from build123d import *

# Parameters (mm, degrees)
BOSS_EXTRUDE4_DEPTH = 5
SKETCH10_R          = 2.5
CUT_EXTRUDE3_DEPTH  = 5


with BuildPart() as part:
    # Sketch9 → Boss-Extrude4 (new body)
    with BuildSketch(Plane.XY):
        with BuildLine():
            add(Edge.make_bspline(
                [(0, 26.124355653), (3.884864274, 23.788582221), (-1.912523876, 17.903903592), (4.641256317, 17.321404385)],
                knots=[0, 0, 0, 0, 1, 1, 1, 1], degree=3))
            add(Edge.make_bspline(
                [(13.062177826, 22.624355653), (8.529899959, 22.54394866), (10.608246058, 14.5489734), (4.641256317, 17.321404385)],
                knots=[0, 0, 0, 0, 1, 1, 1, 1], degree=3))
            add(Edge.make_bspline(
                [(13.062177826, 22.624355653), (15.258682262, 18.659084387), (7.295657534, 16.461497276), (12.680148068, 12.680148068)],
                knots=[0, 0, 0, 0, 1, 1, 1, 1], degree=3))
            add(Edge.make_bspline(
                [(22.624355653, 13.062177826), (18.659084387, 15.258682262), (16.461497276, 7.295657534), (12.680148068, 12.680148068)],
                knots=[0, 0, 0, 0, 1, 1, 1, 1], degree=3))
            add(Edge.make_bspline(
                [(22.624355653, 13.062177826), (22.54394866, 8.529899959), (14.5489734, 10.608246058), (17.321404385, 4.641256317)],
                knots=[0, 0, 0, 0, 1, 1, 1, 1], degree=3))
            add(Edge.make_bspline(
                [(26.124355653, 0), (23.788582221, 3.884864274), (17.903903592, -1.912523876), (17.321404385, 4.641256317)],
                knots=[0, 0, 0, 0, 1, 1, 1, 1], degree=3))
            add(Edge.make_bspline(
                [(26.124355653, 0), (23.788582221, -3.884864274), (17.903903592, 1.912523876), (17.321404385, -4.641256317)],
                knots=[0, 0, 0, 0, 1, 1, 1, 1], degree=3))
            add(Edge.make_bspline(
                [(22.624355653, -13.062177826), (22.54394866, -8.529899959), (14.5489734, -10.608246058), (17.321404385, -4.641256317)],
                knots=[0, 0, 0, 0, 1, 1, 1, 1], degree=3))
            add(Edge.make_bspline(
                [(22.624355653, -13.062177826), (18.659084387, -15.258682262), (16.461497276, -7.295657534), (12.680148068, -12.680148068)],
                knots=[0, 0, 0, 0, 1, 1, 1, 1], degree=3))
            add(Edge.make_bspline(
                [(13.062177826, -22.624355653), (15.258682262, -18.659084387), (7.295657534, -16.461497276), (12.680148068, -12.680148068)],
                knots=[0, 0, 0, 0, 1, 1, 1, 1], degree=3))
            add(Edge.make_bspline(
                [(13.062177826, -22.624355653), (8.529899959, -22.54394866), (10.608246058, -14.5489734), (4.641256317, -17.321404385)],
                knots=[0, 0, 0, 0, 1, 1, 1, 1], degree=3))
            add(Edge.make_bspline(
                [(0, -26.124355653), (3.884864274, -23.788582221), (-1.912523876, -17.903903592), (4.641256317, -17.321404385)],
                knots=[0, 0, 0, 0, 1, 1, 1, 1], degree=3))
            add(Edge.make_bspline(
                [(0, -26.124355653), (-3.884864274, -23.788582221), (1.912523876, -17.903903592), (-4.641256317, -17.321404385)],
                knots=[0, 0, 0, 0, 1, 1, 1, 1], degree=3))
            add(Edge.make_bspline(
                [(-13.062177826, -22.624355653), (-8.529899959, -22.54394866), (-10.608246058, -14.5489734), (-4.641256317, -17.321404385)],
                knots=[0, 0, 0, 0, 1, 1, 1, 1], degree=3))
            add(Edge.make_bspline(
                [(-13.062177826, -22.624355653), (-15.258682262, -18.659084387), (-7.295657534, -16.461497276), (-12.680148068, -12.680148068)],
                knots=[0, 0, 0, 0, 1, 1, 1, 1], degree=3))
            add(Edge.make_bspline(
                [(-22.624355653, -13.062177826), (-18.659084387, -15.258682262), (-16.461497276, -7.295657534), (-12.680148068, -12.680148068)],
                knots=[0, 0, 0, 0, 1, 1, 1, 1], degree=3))
            add(Edge.make_bspline(
                [(-22.624355653, -13.062177826), (-22.54394866, -8.529899959), (-14.5489734, -10.608246058), (-17.321404385, -4.641256317)],
                knots=[0, 0, 0, 0, 1, 1, 1, 1], degree=3))
            add(Edge.make_bspline(
                [(-26.124355653, 0), (-23.788582221, -3.884864274), (-17.903903592, 1.912523876), (-17.321404385, -4.641256317)],
                knots=[0, 0, 0, 0, 1, 1, 1, 1], degree=3))
            add(Edge.make_bspline(
                [(-26.124355653, 0), (-23.788582221, 3.884864274), (-17.903903592, -1.912523876), (-17.321404385, 4.641256317)],
                knots=[0, 0, 0, 0, 1, 1, 1, 1], degree=3))
            add(Edge.make_bspline(
                [(-22.624355653, 13.062177826), (-22.54394866, 8.529899959), (-14.5489734, 10.608246058), (-17.321404385, 4.641256317)],
                knots=[0, 0, 0, 0, 1, 1, 1, 1], degree=3))
            add(Edge.make_bspline(
                [(-22.624355653, 13.062177826), (-18.659084387, 15.258682262), (-16.461497276, 7.295657534), (-12.680148068, 12.680148068)],
                knots=[0, 0, 0, 0, 1, 1, 1, 1], degree=3))
            add(Edge.make_bspline(
                [(-13.062177826, 22.624355653), (-15.258682262, 18.659084387), (-7.295657534, 16.461497276), (-12.680148068, 12.680148068)],
                knots=[0, 0, 0, 0, 1, 1, 1, 1], degree=3))
            add(Edge.make_bspline(
                [(-13.062177826, 22.624355653), (-8.529899959, 22.54394866), (-10.608246058, 14.5489734), (-4.641256317, 17.321404385)],
                knots=[0, 0, 0, 0, 1, 1, 1, 1], degree=3))
            add(Edge.make_bspline(
                [(0, 26.124355653), (-3.884864274, 23.788582221), (1.912523876, 17.903903592), (-4.641256317, 17.321404385)],
                knots=[0, 0, 0, 0, 1, 1, 1, 1], degree=3))
        make_face()
    extrude(amount=BOSS_EXTRUDE4_DEPTH)

    # Sketch10 → Cut-Extrude3 (cut)
    with BuildSketch(Plane.XY.offset(5)):
        Circle(SKETCH10_R)
    extrude(amount=-CUT_EXTRUDE3_DEPTH, mode=Mode.SUBTRACT)


solid = part.part
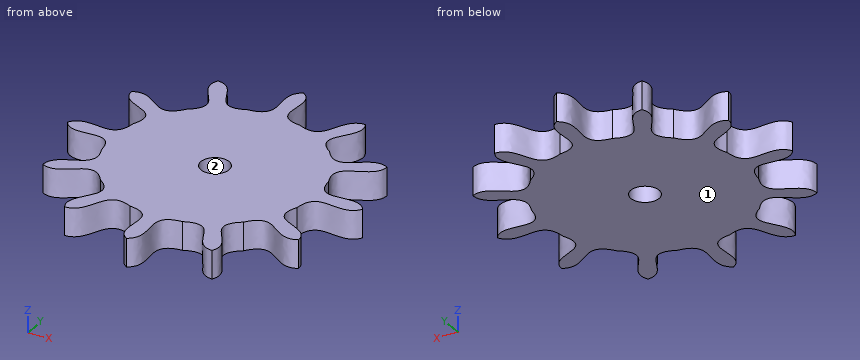
Design review of the part built by this model. Coordinates are the model's own, in mm. Face numbers are marked on the shaded views. Give positions to 0.01 mm unless a question says otherwise; leave off trailing zeros. Answer as a JSON object with one key per item and string values. Group by question number.
1) We need section A-A (y = -12). Count the separate pieces of the cut face and the enclosed holes in it, and give its area (3 significant figures).
2) Clearance check with flat-ended pins moving along their axes: pin 1 Ø1.5 at (x, z) = (12, 1.5) entering from -Y; pin 2 Ø5 at (x, y) = (-16.5, -20) entering from -Z; pin 3 Ø2 at (y, z) = (8.5, 3) entering from -X. State where each tip first meets the part, or that it passes through.
3) Mouldability with a two-part tool opening along Y and no side actions: class the marked faces 1 and 2 as released by +Y, released by -Y, zero draft, split by the parting line, or undercut.
4) For line 1 along Y through (x, z) = (0, 3.85); line 2 along X through (y, z) = (12, 2.4); line 3 along X through (y, z) = (-19.5, 4.1), list the stretches that pass through material, from the lowest coordinate up.
Answer key:
{
 "1": {"separate pieces": "3", "enclosed holes": "0", "area": "176 mm²"},
 "2": {"pin 1": "stops at y = -22.61", "pin 2": "passes through", "pin 3": "stops at x = -19.14"},
 "3": {"face 1": "zero draft", "face 2": "undercut"},
 "4": {"line 1": "y = -26.12 to -2.5, 2.5 to 26.12", "line 2": "x = -22.43 to -18.04, -13.21 to 13.21, 18.04 to 22.43", "line 3": "x = -12.96 to -9.66, -1.35 to 1.35, 9.66 to 12.96"}
}
